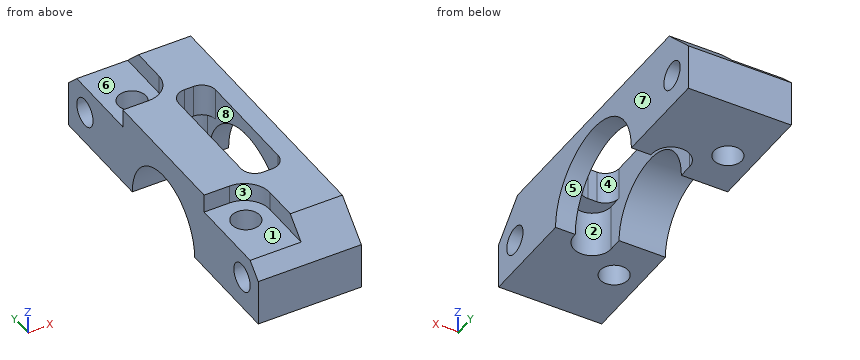
```python
from build123d import *

# Parameters (mm, degrees)
BOSS_EXTRUDE1_DEPTH = 10
BOSS_EXTRUDE2_DEPTH = 12.25
SKETCH3_W           = 22.25
SKETCH3_H           = 8
CUT_EXTRUDE1_DEPTH  = 80
SKETCH8_R           = 3
CUT_EXTRUDE4_DEPTH  = 25
CUT_EXTRUDE2_DEPTH  = 10
SKETCH7_W           = 8
SKETCH7_H           = 29
CUT_EXTRUDE3_DEPTH  = 10
FILLET1_R           = 3
SKETCH19_R          = 3
CUT_EXTRUDE5_DEPTH  = 20
SKETCH21_W          = 4
SKETCH21_H          = 20
CUT_EXTRUDE6_DEPTH  = 11
FILLET2_R           = 5.5
CHAMFER1_SIZE       = 7


with BuildPart() as part:
    # Sketch1 → Boss-Extrude1 (new body)
    with BuildSketch(Plane(origin=(0, 0, 0), x_dir=(0, 0, -1), z_dir=(1, 0, 0))):
        with BuildLine():
            Line((0, 11.5), (0, 35))
            Line((0, 35), (-25, 35))
            Line((-25, 35), (-25, -35))
            Line((-25, -35), (0, -35))
            Line((0, -35), (0, -11.5))
            ThreePointArc((0, -11.5), (-11.5, 0), (0, 11.5))
        make_face()
    extrude(amount=BOSS_EXTRUDE1_DEPTH)

    # Sketch2 → Boss-Extrude2 (add)
    with BuildSketch(Plane(origin=(10, 0, 0), x_dir=(0, 0, -1), z_dir=(1, 0, 0))):
        with BuildLine():
            Line((0, -14), (0, -35))
            Line((0, -35), (-25, -35))
            Line((-25, -35), (-25, 35))
            Line((-25, 35), (0, 35))
            Line((0, 35), (0, 14))
            ThreePointArc((0, 14), (-14, 0), (0, -14))
        make_face()
    extrude(amount=BOSS_EXTRUDE2_DEPTH)

    # Sketch3 → Cut-Extrude1 (cut)
    with BuildSketch(Plane.XZ.offset(35)):
        with Locations((11.125, 21)):
            Rectangle(SKETCH3_W, SKETCH3_H)
    extrude(amount=-CUT_EXTRUDE1_DEPTH, mode=Mode.SUBTRACT)

    # Sketch8 → Cut-Extrude4 (cut)
    with BuildSketch(Plane(origin=(22.25, 0, 0), x_dir=(0, 0, -1), z_dir=(1, 0, 0))):
        with Locations((-7, -29)):
            Circle(SKETCH8_R)
        with Locations((-7, 29)):
            Circle(SKETCH8_R)
    extrude(amount=-CUT_EXTRUDE4_DEPTH, mode=Mode.SUBTRACT)

    # Sketch6 → Cut-Extrude2 (cut)
    with BuildSketch(Plane(origin=(0, 0, 0), x_dir=(-1, 0, 0), z_dir=(0, 0, -1))):
        with BuildLine():
            Line((-18, -14.5), (-18, 14.5))
            ThreePointArc((-18, 14.5), (-14, 18.5), (-10, 14.5))
            Line((-10, 14.5), (-10, -14.5))
            ThreePointArc((-10, -14.5), (-14, -18.5), (-18, -14.5))
        make_face()
    extrude(amount=-CUT_EXTRUDE2_DEPTH, mode=Mode.SUBTRACT)

    # Sketch7 → Cut-Extrude3 (cut)
    with BuildSketch(Plane(origin=(0, 0, 10), x_dir=(-1, 0, 0), z_dir=(0, 0, -1))):
        with Locations((-14, 0)):
            Rectangle(SKETCH7_W, SKETCH7_H)
    extrude(amount=-CUT_EXTRUDE3_DEPTH, mode=Mode.SUBTRACT)

    # Fillet1
    fillet1_edges = [part.edges().sort_by_distance(p)[0] for p in [
        (18, 14.5, 13.5),
        (18, -14.5, 13.5),
        (10, 14.5, 13.5),
        (10, -14.5, 13.5),
    ]]
    fillet(fillet1_edges, radius=FILLET1_R)

    # Sketch19 → Cut-Extrude5 (cut)
    with BuildSketch(Plane(origin=(0, 0, 0), x_dir=(-1, 0, 0), z_dir=(0, 0, -1))):
        with Locations(Location((-5.5, -21, 0), (0, 0, 90))):
            Circle(SKETCH19_R)
        with Locations(Location((-5.5, 21, 0), (0, 0, 90))):
            Circle(SKETCH19_R)
    extrude(amount=-CUT_EXTRUDE5_DEPTH, mode=Mode.SUBTRACT)

    # Sketch21 → Cut-Extrude6 (cut)
    with BuildSketch(Plane.ZY):
        with Locations((15, -25)):
            Rectangle(SKETCH21_W, SKETCH21_H)
        with Locations((15, 25)):
            Rectangle(SKETCH21_W, SKETCH21_H)
    extrude(amount=-CUT_EXTRUDE6_DEPTH, mode=Mode.SUBTRACT)

    # Fillet2
    fillet2_edges = [part.edges().sort_by_distance(p)[0] for p in [
        (11, -15, 15),
        (11, 15, 15),
    ]]
    fillet(fillet2_edges, radius=FILLET2_R)

    # Chamfer1
    chamfer1_edges = [part.edges().sort_by_distance(p)[0] for p in [
        (16.625, -35, 17),
        (16.625, 35, 17),
    ]]
    chamfer(chamfer1_edges, length=CHAMFER1_SIZE)


solid = part.part
```
Work out the finished part from the listing and answer in its coordinate system (mm). Face numbers are marked on the shaded views. A direction names the side the tool comes from. Round coordinates to 2 decimals unless told otherwise and drop trailing zeros. Write each loop counter-clockwise with the first axis right and the second up, starting at its lowest first coordinate (ties: lowest second). Pieces come first, ordered by that corner, then holes. Notation, with made-up numbers: (-7, 41.5) - (8, 41.5) arc R26 ccw to (8, 57.5) - close; hole circle Ø8 at (14.5, 33.25). An arc over 180 degrees is marked (long way). Return JSON: item names as keys, results as strings. Group by question number.
Q1. Find the intervals of material crossed by L1, parallel to X at y = 21, z = 5.5; L2, parallel to Y at x = 19.75, z = 9; L3, parallel to Y at x = 3.5, z = 1.25, in increasing order.
Q2. The part is cut by section C-C on z = 8. Write down the section's boundary in (x, y).
Q3. The part is cut by section D-D on x = 3.5. Write down the section's boundary in (y, z).
Q4. The mould has two halves that part along X. Classify the marked faces 1, 2 and 3: released by +X, released by -X, zero draft, split by the parting line, or undercut.
Q5. The part is cut by section A-A on x = 19.25. Write down the section's boundary in (y, z).
Q6. For the marked faces 4, 5, 6, 7 and 8, determine the directions among +Z, -Z, +X, -X, +Y, -Y from which every point of the face is accessible in a straight line to the end or side of a thin tool.
Q7. Each of these flat-tipped pins is pushed along its axis until it touches: pin 1 Ø5 at (x, y) = (5.5, 21) entering from +Z; pin 2 Ø7 at (x, y) = (5.5, -21) entering from -Z; pin 3 Ø3 at (x, z) = (2.5, 15) entering from +Y; pin 4 Ø2 at (x, y) = (12, -15.5) entering from -Z. Where does it stop, or does it pass through?
Q8. The part is cut by section B-B on y = 0. Write down the section's boundary in (x, z), then the cut area to 4 significant figures.
Solved:
{
 "1": {"L1": "0 to 2.5, 8.5 to 22.25", "L2": "-35 to -31.24, -26.76 to -10.72, 10.72 to 26.76, 31.24 to 35", "L3": "-35 to -23.24, -18.76 to -11.43, 11.43 to 18.76, 23.24 to 35"},
 "2": {"outline": "(0, -35) - (22.25, -35) - (22.25, -31.83) - (0, -31.83) - close; (0, -26.17) - (22.25, -26.17) - (22.25, -11.49) - (18, -11.49) - (18, -14.5) arc R4 cw to (10, -14.5) - (10, -8.26) - (0, -8.26) - close; (0, 8.26) - (10, 8.26) - (10, 14.5) arc R4 cw to (18, 14.5) - (18, 11.49) - (22.25, 11.49) - (22.25, 26.17) - (0, 26.17) - close; (0, 31.83) - (22.25, 31.83) - (22.25, 35) - (0, 35) - close; hole circle Ø6 at (5.5, -21); hole circle Ø6 at (5.5, 21)"},
 "3": {"outline": "(-35, 0) - (-23.24, 0) - (-23.24, 13) - (-32, 13) - (-35, 10) - close; (-18.76, 0) - (-11.5, 0) arc R11.5 cw to (11.5, 0) - (18.76, 0) - (18.76, 13) - (15, 13) - (15, 17) - (-15, 17) - (-15, 13) - (-18.76, 13) - close; (23.24, 0) - (35, 0) - (35, 10) - (32, 13) - (23.24, 13) - close; hole circle Ø6 at (-29, 7); hole circle Ø6 at (29, 7)"},
 "4": {"face 1": "zero draft", "face 2": "undercut", "face 3": "released by -X"},
 "5": {"outline": "(-35, 0) - (-14, 0) arc R14 cw to (14, 0) - (35, 0) - (35, 10) - (28, 17) - (-28, 17) - (-35, 10) - close; hole circle Ø6 at (-29, 7); hole circle Ø6 at (29, 7)"},
 "6": {"face 4": "+Z, -Z", "face 5": "-Z, +X", "face 6": "+Z, -X, +Y", "face 7": "+Z, -Z, +X, +Y, -Y", "face 8": "-Z"},
 "7": {"pin 1": "through", "pin 2": "z = 0", "pin 3": "y = 15", "pin 4": "z = 10"},
 "8": {"outline": "(0, 11.5) - (10, 11.5) - (10, 17) - (0, 17) - close; (18, 14) - (22.25, 14) - (22.25, 17) - (18, 17) - close", "area": "67.75 mm²"}
}
